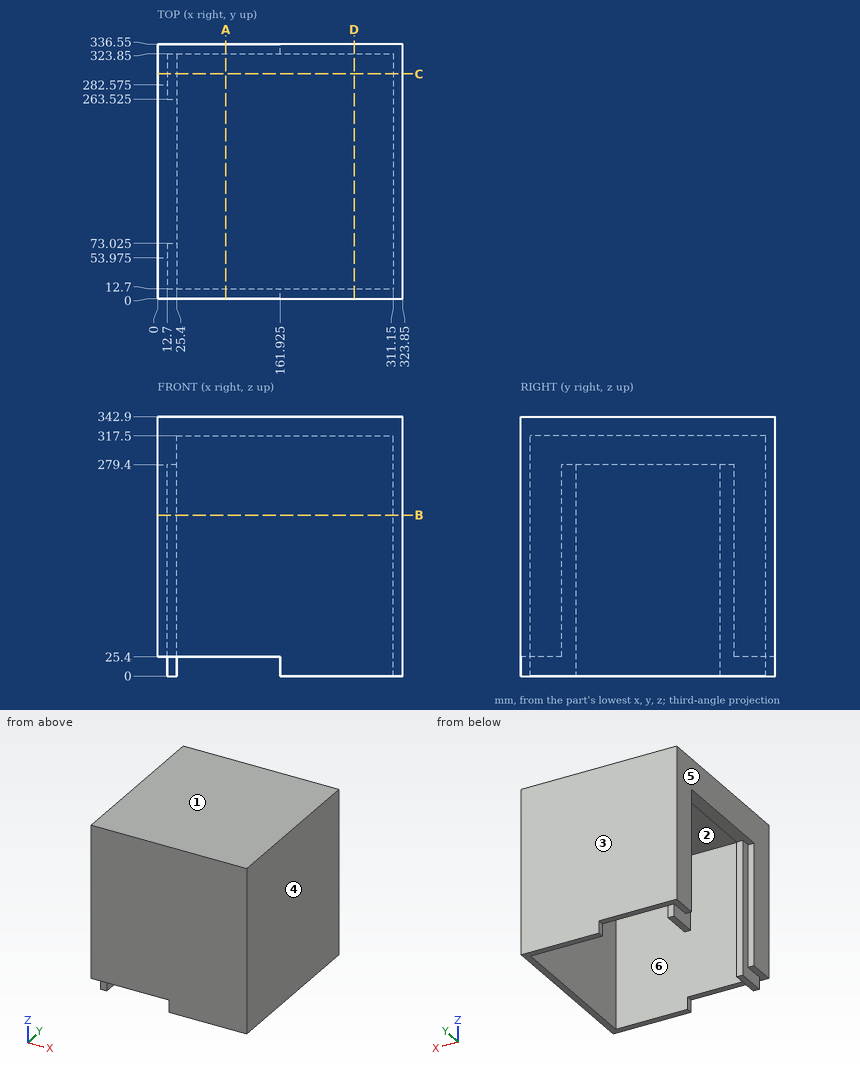
For this review, use the dimensioned drawing (mm, ordinates from the lowest corner) and the shaded views. A direction names the side the tool comes from. Coordinates: 2 decimals unless noted, no trailing zeros. Loops run counter-clockwise (first coordinate to the right, second up) from the corner with the lowest first, then second, coordinate; pieces in that order, holes last. Notation, with made-up numbers: (26, 59.5) -> (45, 59.5) arc R25 ccw to (45, 78.5) -> close; hole circle Ø6 at (-0.5, 70). An arc over 180 degrees is marked (long way). Use a Markdown table: item, result. Add a question column.
1. To check wall thickness, follow line 1 (Y direction, x = 50, z = 288.5); line 2 (X direction, y = 34, z = 201); line 3 (Y direction, x = 21.5, z = 95) (3 decimals). State the ranges of each line that lie inside material, in increasing order.
2. Add section B-B on z = 212.5. Write out the cut boundary in (x, y) (3 decimals), plus the area to 3 significant figures.
3. Machinability: for the marked faces 1 and 2, which of the approach directions +Z, -Z, +X, -X, +Y, -Y give a long, thin tool a straight path to every point of the face, cutting with its end or side? Answer none if there is none.
4. Draft analysis for pull direction X (two halves, no side actions). For the marked faces 3, 4, 5 and 6, state which applies: pulls with the +X half, pulls with the -X half, needs draft (parallel to the pull), parting line crosses it, or undercut.
5. Clearance check with flat-ended pins moving along their axes: pin 1 Ø10 at (x, y) = (193, 61) entering from -Z; pin 2 Ø12 at (y, z) = (91.5, 121.5) entering from -X; pin 3 Ø10 at (y, z) = (332, 8.5) entering from -X (3 decimals). State where each tip first meets the part, or that it passes through.
6. Add section A-A on x = 90. Write out the cut boundary in (y, z), plus the area to 3 significant figures.
7. Add section D-D on x = 259.5. Write out the cut boundary in (y, z).
8. Add section C-C on y = 297. Write out the cut boundary in (x, z).
Returned:
| question | item | result |
|---|---|---|
| 1 | line 1 | y = 0 to 12.7, 323.85 to 336.55 |
| 1 | line 2 | x = 0 to 25.4, 311.15 to 323.85 |
| 1 | line 3 | y = 0 to 73.025, 263.525 to 336.55 |
| 2 | outline | (0, 0) -> (323.85, 0) -> (323.85, 336.55) -> (0, 336.55) -> (0, 282.575) -> (12.7, 282.575) -> (12.7, 263.525) -> (25.4, 263.525) -> (25.4, 323.85) -> (311.15, 323.85) -> (311.15, 12.7) -> (25.4, 12.7) -> (25.4, 73.025) -> (12.7, 73.025) -> (12.7, 53.975) -> (0, 53.975) -> close |
| 2 | area | 14,800 mm² |
| 3 | face 1 | +Z, +X, -X, +Y, -Y |
| 3 | face 2 | -Z |
| 4 | face 3 | needs draft |
| 4 | face 4 | pulls with the +X half |
| 4 | face 5 | pulls with the -X half |
| 4 | face 6 | undercut |
| 5 | pin 1 | stops at z = 317.5 |
| 5 | pin 2 | stops at x = 311.15 |
| 5 | pin 3 | stops at x = 161.925 |
| 6 | outline | (0, 25.4) -> (12.7, 25.4) -> (12.7, 317.5) -> (323.85, 317.5) -> (323.85, 25.4) -> (336.55, 25.4) -> (336.55, 342.9) -> (0, 342.9) -> close |
| 6 | area | 16,000 mm² |
| 7 | outline | (0, 0) -> (12.7, 0) -> (12.7, 317.5) -> (323.85, 317.5) -> (323.85, 0) -> (336.55, 0) -> (336.55, 342.9) -> (0, 342.9) -> close |
| 8 | outline | (0, 25.4) -> (12.7, 25.4) -> (12.7, 0) -> (25.4, 0) -> (25.4, 317.5) -> (311.15, 317.5) -> (311.15, 0) -> (323.85, 0) -> (323.85, 342.9) -> (0, 342.9) -> close |
